from build123d import *

# Parameters (mm, degrees)
BOSS_EXTRUDE1_DEPTH = 9.55
CHAMFER1_SIZE       = 3
CUT_EXTRUDE1_REACH  = 630.926
SKETCH2_R           = 2.565
SKETCH2_R_2         = 3.445
SKETCH2_R_3         = 2.795
SKETCH2_R_4         = 2.48
SKETCH2_R_5         = 1.385
SKETCH3_R           = 4.61
CUT_EXTRUDE2_DEPTH  = 5.2
SKETCH4_R           = 3.98
CUT_EXTRUDE3_DEPTH  = 4.54
SKETCH5_R           = 3.445
CUT_EXTRUDE4_DEPTH  = 7.68
SKETCH6_R           = 4
SKETCH6_R_2         = 2.565
BOSS_EXTRUDE2_DEPTH = 2.5
SKETCH7_R           = 2.065
CUT_EXTRUDE5_DEPTH  = 18.99
SKETCH8_R           = 2.065
CUT_EXTRUDE6_DEPTH  = 18.7


with BuildPart() as part:
    # Sketch1 → Boss-Extrude1 (new body)
    with BuildSketch(Plane(origin=(0, 0, 0), x_dir=(1, 0, 0), z_dir=(0, 1, 0))):
        Polygon((532.64, 0), (621.59, 0), (621.59, -95.3), (0, -95.3), (0, 0), (462.84, 0), (462.84, -9.5), (532.64, -9.5), align=None)
    extrude(amount=BOSS_EXTRUDE1_DEPTH)

    # Chamfer1
    chamfer1_edges = [part.edges().sort_by_distance(p)[0] for p in [
        (577.115, 9.55, 0),
        (231.42, 9.55, 0),
    ]]
    chamfer(chamfer1_edges, length=CHAMFER1_SIZE)

    # Sketch2 → Cut-Extrude1 (cut, up to next)
    with BuildSketch(Plane(origin=(0, 9.55, 0), x_dir=(-1, 0, 0), z_dir=(0, 1, 0)), mode=Mode.PRIVATE) as cut_extrude1_sk1:
        with Locations(Location((-611.995, 63.695, 0), (0, 0, 90))):
            Circle(SKETCH2_R)
    cut_extrude1_tool1 = extrude(cut_extrude1_sk1.sketch, amount=-CUT_EXTRUDE1_REACH, mode=Mode.PRIVATE) & part.part
    # Sketch2 → Cut-Extrude1 (cut, up to next)
    with BuildSketch(Plane(origin=(0, 9.55, 0), x_dir=(-1, 0, 0), z_dir=(0, 1, 0)), mode=Mode.PRIVATE) as cut_extrude1_sk2:
        with Locations(Location((-554.785, 63.695, 0), (0, 0, 90))):
            Circle(SKETCH2_R_2)
    cut_extrude1_tool2 = extrude(cut_extrude1_sk2.sketch, amount=-CUT_EXTRUDE1_REACH, mode=Mode.PRIVATE) & part.part
    # Sketch2 → Cut-Extrude1 (cut, up to next)
    with BuildSketch(Plane(origin=(0, 9.55, 0), x_dir=(-1, 0, 0), z_dir=(0, 1, 0)), mode=Mode.PRIVATE) as cut_extrude1_sk3:
        with Locations(Location((-6.42, 19.16, 0), (0, 0, 90))):
            Circle(SKETCH2_R_3)
    cut_extrude1_tool3 = extrude(cut_extrude1_sk3.sketch, amount=-CUT_EXTRUDE1_REACH, mode=Mode.PRIVATE) & part.part
    # Sketch2 → Cut-Extrude1 (cut, up to next)
    with BuildSketch(Plane(origin=(0, 9.55, 0), x_dir=(-1, 0, 0), z_dir=(0, 1, 0)), mode=Mode.PRIVATE) as cut_extrude1_sk4:
        with Locations(Location((-6.42, 73.05, 0), (0, 0, 90))):
            Circle(SKETCH2_R_3)
    cut_extrude1_tool4 = extrude(cut_extrude1_sk4.sketch, amount=-CUT_EXTRUDE1_REACH, mode=Mode.PRIVATE) & part.part
    # Sketch2 → Cut-Extrude1 (cut, up to next)
    with BuildSketch(Plane(origin=(0, 9.55, 0), x_dir=(-1, 0, 0), z_dir=(0, 1, 0)), mode=Mode.PRIVATE) as cut_extrude1_sk5:
        with Locations(Location((-575.61, 76.28, 0), (0, 0, 90))):
            Circle(SKETCH2_R_4)
    cut_extrude1_tool5 = extrude(cut_extrude1_sk5.sketch, amount=-CUT_EXTRUDE1_REACH, mode=Mode.PRIVATE) & part.part
    # Sketch2 → Cut-Extrude1 (cut, up to next)
    with BuildSketch(Plane(origin=(0, 9.55, 0), x_dir=(-1, 0, 0), z_dir=(0, 1, 0)), mode=Mode.PRIVATE) as cut_extrude1_sk6:
        with Locations(Location((-575.61, 31.84, 0), (0, 0, 90))):
            Circle(SKETCH2_R_4)
    cut_extrude1_tool6 = extrude(cut_extrude1_sk6.sketch, amount=-CUT_EXTRUDE1_REACH, mode=Mode.PRIVATE) & part.part
    # Sketch2 → Cut-Extrude1 (cut, up to next)
    with BuildSketch(Plane(origin=(0, 9.55, 0), x_dir=(-1, 0, 0), z_dir=(0, 1, 0)), mode=Mode.PRIVATE) as cut_extrude1_sk7:
        with Locations(Location((-539.07, 73.05, 0), (0, 0, 90))):
            Circle(SKETCH2_R_3)
    cut_extrude1_tool7 = extrude(cut_extrude1_sk7.sketch, amount=-CUT_EXTRUDE1_REACH, mode=Mode.PRIVATE) & part.part
    # Sketch2 → Cut-Extrude1 (cut, up to next)
    with BuildSketch(Plane(origin=(0, 9.55, 0), x_dir=(-1, 0, 0), z_dir=(0, 1, 0)), mode=Mode.PRIVATE) as cut_extrude1_sk8:
        with Locations(Location((-539.07, 19.16, 0), (0, 0, 90))):
            Circle(SKETCH2_R_3)
    cut_extrude1_tool8 = extrude(cut_extrude1_sk8.sketch, amount=-CUT_EXTRUDE1_REACH, mode=Mode.PRIVATE) & part.part
    # Sketch2 → Cut-Extrude1 (cut, up to next)
    with BuildSketch(Plane(origin=(0, 9.55, 0), x_dir=(-1, 0, 0), z_dir=(0, 1, 0)), mode=Mode.PRIVATE) as cut_extrude1_sk9:
        with Locations(Location((-19.135, 63.695, 0), (0, 0, 90))):
            Circle(SKETCH2_R)
    cut_extrude1_tool9 = extrude(cut_extrude1_sk9.sketch, amount=-CUT_EXTRUDE1_REACH, mode=Mode.PRIVATE) & part.part
    # Sketch2 → Cut-Extrude1 (cut, up to next)
    with BuildSketch(Plane(origin=(0, 9.55, 0), x_dir=(-1, 0, 0), z_dir=(0, 1, 0)), mode=Mode.PRIVATE) as cut_extrude1_sk10:
        with Locations(Location((-76.345, 63.695, 0), (0, 0, 90))):
            Circle(SKETCH2_R)
    cut_extrude1_tool10 = extrude(cut_extrude1_sk10.sketch, amount=-CUT_EXTRUDE1_REACH, mode=Mode.PRIVATE) & part.part
    # Sketch2 → Cut-Extrude1 (cut, up to next)
    with BuildSketch(Plane(origin=(0, 9.55, 0), x_dir=(-1, 0, 0), z_dir=(0, 1, 0)), mode=Mode.PRIVATE) as cut_extrude1_sk11:
        with Locations(Location((-602.545, 9.5, 0), (0, 0, 90))):
            Circle(SKETCH2_R_5)
    cut_extrude1_tool11 = extrude(cut_extrude1_sk11.sketch, amount=-CUT_EXTRUDE1_REACH, mode=Mode.PRIVATE) & part.part
    add(cut_extrude1_tool1.solids().sort_by_distance((611.995, 9.55, 63.695))[0], mode=Mode.SUBTRACT)
    add(cut_extrude1_tool2.solids().sort_by_distance((554.785, 9.55, 63.695))[0], mode=Mode.SUBTRACT)
    add(cut_extrude1_tool3.solids().sort_by_distance((6.42, 9.55, 19.16))[0], mode=Mode.SUBTRACT)
    add(cut_extrude1_tool4.solids().sort_by_distance((6.42, 9.55, 73.05))[0], mode=Mode.SUBTRACT)
    add(cut_extrude1_tool5.solids().sort_by_distance((575.61, 9.55, 76.28))[0], mode=Mode.SUBTRACT)
    add(cut_extrude1_tool6.solids().sort_by_distance((575.61, 9.55, 31.84))[0], mode=Mode.SUBTRACT)
    add(cut_extrude1_tool7.solids().sort_by_distance((539.07, 9.55, 73.05))[0], mode=Mode.SUBTRACT)
    add(cut_extrude1_tool8.solids().sort_by_distance((539.07, 9.55, 19.16))[0], mode=Mode.SUBTRACT)
    add(cut_extrude1_tool9.solids().sort_by_distance((19.135, 9.55, 63.695))[0], mode=Mode.SUBTRACT)
    add(cut_extrude1_tool10.solids().sort_by_distance((76.345, 9.55, 63.695))[0], mode=Mode.SUBTRACT)
    add(cut_extrude1_tool11.solids().sort_by_distance((602.545, 9.55, 9.5))[0], mode=Mode.SUBTRACT)

    # Sketch3 → Cut-Extrude2 (cut)
    with BuildSketch(Plane(origin=(0, 9.55, 0), x_dir=(-1, 0, 0), z_dir=(0, 1, 0))):
        with Locations(Location((-6.42, 19.16, 0), (0, 0, 90))):
            Circle(SKETCH3_R)
        with Locations(Location((-6.42, 73.05, 0), (0, 0, 90))):
            Circle(SKETCH3_R)
        with Locations(Location((-539.07, 19.16, 0), (0, 0, 90))):
            Circle(SKETCH3_R)
        with Locations(Location((-539.07, 73.05, 0), (0, 0, 90))):
            Circle(SKETCH3_R)
    extrude(amount=-CUT_EXTRUDE2_DEPTH, mode=Mode.SUBTRACT)

    # Sketch4 → Cut-Extrude3 (cut)
    with BuildSketch(Plane(origin=(0, 9.55, 0), x_dir=(-1, 0, 0), z_dir=(0, 1, 0))):
        with Locations(Location((-575.61, 31.84, 0), (0, 0, 90))):
            Circle(SKETCH4_R)
        with Locations(Location((-575.61, 76.28, 0), (0, 0, 90))):
            Circle(SKETCH4_R)
    extrude(amount=-CUT_EXTRUDE3_DEPTH, mode=Mode.SUBTRACT)

    # Sketch5 → Cut-Extrude4 (cut)
    with BuildSketch(Plane(origin=(0, 9.55, 0), x_dir=(-1, 0, 0), z_dir=(0, 1, 0))):
        with Locations(Location((-611.995, 63.695, 0), (0, 0, 90))):
            Circle(SKETCH5_R)
        with Locations(Location((-76.345, 63.695, 0), (0, 0, 90))):
            Circle(SKETCH5_R)
        with Locations(Location((-19.135, 63.695, 0), (0, 0, 90))):
            Circle(SKETCH5_R)
    extrude(amount=-CUT_EXTRUDE4_DEPTH, mode=Mode.SUBTRACT)

    # Sketch6 → Boss-Extrude2 (add)
    with BuildSketch(Plane.XZ):
        with Locations(Location((611.995, 63.695, 0), (0, 0, 90))):
            Circle(SKETCH6_R)
        with Locations(Location((611.995, 63.695, 0), (0, 0, 90))):
            Circle(SKETCH6_R_2, mode=Mode.SUBTRACT)
        with Locations(Location((76.345, 63.695, 0), (0, 0, 90))):
            Circle(SKETCH6_R)
        with Locations(Location((76.345, 63.695, 0), (0, 0, 90))):
            Circle(SKETCH6_R_2, mode=Mode.SUBTRACT)
        with Locations(Location((19.135, 63.695, 0), (0, 0, 90))):
            Circle(SKETCH6_R)
        with Locations(Location((19.135, 63.695, 0), (0, 0, 90))):
            Circle(SKETCH6_R_2, mode=Mode.SUBTRACT)
    extrude(amount=BOSS_EXTRUDE2_DEPTH)

    # Sketch7 → Cut-Extrude5 (cut)
    with BuildSketch(Plane(origin=(0, 0, 9.5), x_dir=(-1, 0, 0), z_dir=(0, 0, -1))):
        with Locations((-507.305, 4.775)):
            Circle(SKETCH7_R)
        with Locations((-475.355, 4.775)):
            Circle(SKETCH7_R)
    extrude(amount=-CUT_EXTRUDE5_DEPTH, mode=Mode.SUBTRACT)

    # Sketch8 → Cut-Extrude6 (cut)
    with BuildSketch(Plane(origin=(621.59, 0, 0), x_dir=(0, 0, -1), z_dir=(1, 0, 0))):
        with Locations((-31.685, 4.775)):
            Circle(SKETCH8_R)
        with Locations((-37.755, 4.775)):
            Circle(SKETCH8_R)
        with Locations((-69.865, 4.775)):
            Circle(SKETCH8_R)
        with Locations((-75.935, 4.775)):
            Circle(SKETCH8_R)
    extrude(amount=-CUT_EXTRUDE6_DEPTH, mode=Mode.SUBTRACT)


solid = part.part
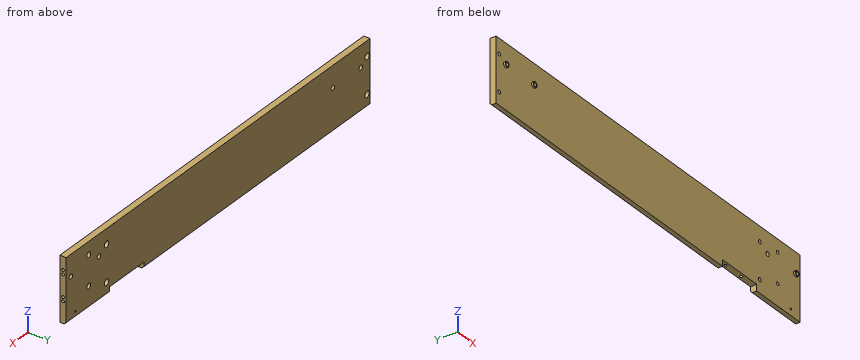
CAD build for the part. Positions are in the model's coordinates, mm. Give positions to 0.01 mm unless a question says otherwise; leave off trailing zeros. Write each loop counter-clockwise with the first axis right and the second up, starting at its lowest first coordinate (ties: lowest second). Pieces come first, ordered by that corner, then holes. Notation, with made-up numbers: M -35,-5 L -31,-5 A18 cw -31,16 Z; hole C 27,17.25 d5. An arc over 180 degrees is marked long. Put each result on its own line as item: value. Start each with the question number.
(1) Probe L1, parallel to X at y = 6.6, z = 19.16; L2, parallel to X at y = 2.5, z = 62.5; L3, parallel to Y at x = 529, z = 48.5. List the from-to ranges inside material, lowest first.
(2) Band-saw the part on A-A, the plane x = 139.5. Write the cut outline in (y, z), and give its area (3 significant figures).
(3) Flat gauge pins, fed straight in: pin 1 Ø6 at (x, z) = (19.135, 63.695) entering from +Y; pin 2 Ø3.5 at (y, z) = (4.775, 69.865) entering from -X; pin 3 Ø7.5 at (x, z) = (539.07, 19.16) entering from +Y; pin 4 Ø1.5 at (x, z) = (367.5, 21) entering from -Y. Where does each tip first touch, or does it go through?
Response values:
1. L1: x = 0 to 1.81, 11.03 to 474.39, 476.32 to 506.34, 508.27 to 534.46, 543.68 to 621.59
1. L2: x = 0 to 15.9, 22.37 to 73.11, 79.58 to 551.55, 558.02 to 608.76, 615.23 to 621.59
1. L3: y = 0 to 9.55
2. outline: M 0,0 L 6.55,0 L 9.55,3 L 9.55,95.3 L 0,95.3 Z
2. area: 906 mm2
3. pin 1: stops at y = 1.87
3. pin 2: stops at x = 0
3. pin 3: stops at y = 4.35
3. pin 4: stops at y = 0
